Can you work these out from the model? Positions are in its coordinate system, mm. Face numbers are marked on the shaded views. A direction names the side the tool comes from. Round coordinates to 2 decimals unless told otherwise and drop trailing zeros. Order: outer loops, then holes, each group sorted by start corner. A loop starts at its lowest first (then second) coordinate and runs counter-clockwise, first axis right, second up. Notation, with made-up numbers: (66.25, -19) -> (87.25, -19) arc R12 cw to (87.25, 4) -> close; hole circle Ø1 at (35, 34). An arc over 180 degrees is marked (long way). Use a Markdown table: item, result. Add a question column.
Q1. If we section it at A-A on z = 10.25: List the corners of the cut face in (x, y) for me (3 decimals), plus the area to 3 significant figures.
Q2. For the marked faces 1 and 2, which set-ups out of +Z, -Z, +X, -X, +Y, -Y let a thin tool reach every point of the face, with its end or its side?
Q3. If we section it at D-D on y = -10: List the corners of the cut face in (x, z) for me.
Q4. If we section it at B-B on x = 0: List the corners of the cut face in (y, z) for me (3 decimals).
Q5. If we section it at C-C on y = -4.5: List the corners of the cut face in (x, z) for me, plus the area to 3 significant figures.
Q6. We'd pull the mould along X, two halves only. Please class the marked faces 3, 4, 5 and 6: +X half, -X half, draft (parallel to the pull), parting line (faces both ways), or undercut.
Q7. I'm going to push flat-ended pins straight in: pin 1 Ø2 at (x, z) = (8.5, 19) entering from +Y; pin 2 Ø3 at (y, z) = (7, 10) entering from -X; pin 3 Ø6 at (x, z) = (11.5, 4.5) entering from +Y. Where does each tip first touch, or does it pass through?
Q8. I need wall thicknesses on line 1 along Y through (x, z) = (-0.5, 6.25); line 2 along X through (y, z) = (5, 2); line 3 along X through (y, z) = (-3, 5.25). Which ranges of each line are inside material? Lowest first, please. Write a range as [from, to].
```python
from build123d import *

# Parameters (mm, degrees)
SKETCH1_R           = 15.875
BOSS_EXTRUDE1_DEPTH = 25.4
CUT_EXTRUDE1_DEPTH  = 26.4


with BuildPart() as part:
    # Sketch1 → Boss-Extrude1 (new body)
    with BuildSketch(Plane.XY):
        Circle(SKETCH1_R)
    extrude(amount=BOSS_EXTRUDE1_DEPTH)

    # Sketch3 → Cut-Extrude1 (cut, through all)
    with BuildSketch(Plane.XY.offset(25.4)):
        Polygon((6.35, 0), (3.175, 5.499261314), (-3.175, 5.499261314), (-6.35, 0), (-3.175, -5.499261314), (3.175, -5.499261314), align=None)
    extrude(amount=-CUT_EXTRUDE1_DEPTH, mode=Mode.SUBTRACT)


solid = part.part
```
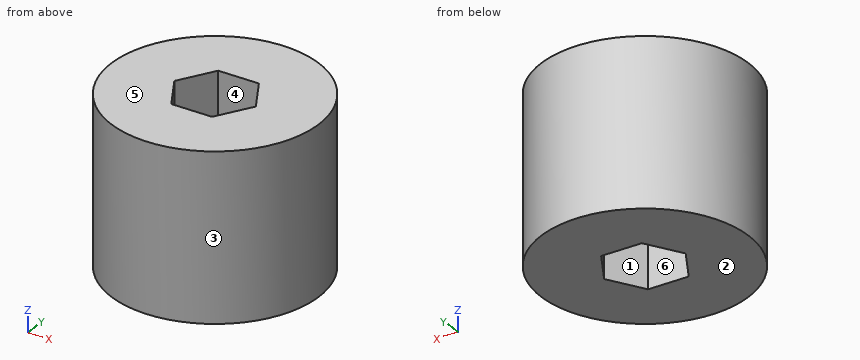
Answer below:
| question | item | result |
|---|---|---|
| 1 | outline | circle Ø31.75 at (0, 0); hole (-6.35, 0) -> (-3.175, -5.499) -> (3.175, -5.499) -> (6.35, 0) -> (3.175, 5.499) -> (-3.175, 5.499) -> close |
| 1 | area | 687 mm² |
| 2 | face 1 | +Z, -Z |
| 2 | face 2 | -Z, +X, -X, +Y, -Y |
| 3 | outline | (-12.33, 0) -> (12.33, 0) -> (12.33, 25.4) -> (-12.33, 25.4) -> close |
| 4 | outline | (-15.875, 0) -> (-5.499, 0) -> (-5.499, 25.4) -> (-15.875, 25.4) -> close; (5.499, 0) -> (15.875, 0) -> (15.875, 25.4) -> (5.499, 25.4) -> close |
| 5 | outline | (-15.22, 0) -> (-3.75, 0) -> (-3.75, 25.4) -> (-15.22, 25.4) -> close; (3.75, 0) -> (15.22, 0) -> (15.22, 25.4) -> (3.75, 25.4) -> close |
| 5 | area | 583 mm² |
| 6 | face 3 | parting line |
| 6 | face 4 | undercut |
| 6 | face 5 | draft |
| 6 | face 6 | undercut |
| 7 | pin 1 | y = 13.99 |
| 7 | pin 2 | x = -14.89 |
| 7 | pin 3 | y = 13.41 |
| 8 | line 1 | [-15.87, -5.5], [5.5, 15.87] |
| 8 | line 2 | [-15.07, -3.46], [3.46, 15.07] |
| 8 | line 3 | [-15.59, -4.62], [4.62, 15.59] |
